Input: part model. Units: mm. Frame: model coordinates. Round coordinates to 2 decimals unless told otherwise and drop trailing zeros. Loops run counter-clockwise (first coordinate to the right, second up) from the corner with the lowest first, then second, coordinate; pieces in that order, holes last. Notation, with made-up numbers: (-10, -21) -> (45, -21) arc R33 ccw to (45, 16) -> close; hole circle Ø11 at (-39.75, 20.25). An arc over 180 degrees is marked (long way). Answer in a Markdown table with one row per item. Add a question column.
Q1. Ray query, L1, parallel to X at y = 3, z = 74 (3 decimals); L2, parallel to X at y = 4.25, z = 20; L3, parallel to X at y = 3.75, z = 33. Return the intervals inside material, ascending. Write a range as from..to.
Q2. Section A-A, the plane y = 3.75. Give the number of separate pieces and of enclosed holes in the cut face, and give its area (3 significant figures).
Q3. Section B-B, the plane z = 13. Output: boundary loops of the cut face in (x, y).
Q4. Section C-C, the plane x = 11. Output: boundary loops of the cut face in (y, z), and give its area (3 significant figures).
Q5. Section D-D, the plane z = -63. Output: boundary loops of the cut face in (x, y).
Q6. Pin query (flat end, axial travel): pin 1 (8 mm diameter, centred on x = -17, z = 57, fed in from -Y); pin 2 (2 mm diameter, centred on x = -19.05, z = -75, fed in from +Y); pin 3 (2 mm diameter, centred on y = 5.5, z = 18, fed in from +X); pin 4 (1 mm diameter, centred on y = 3, z = -15.5, fed in from -X). Return the tip coordinate at first contact, or that it passes through.
```python
from build123d import *

# Parameters (mm, degrees)
SKETCH2_R             = 90
EXTRUDE1_DEPTH        = 7
SKETCH3_R             = 8
CUT_EXTRUDE1_DEPTH    = 8
M3X0_5_TAPPED_HOLE1_D = 2.5
CIRPATTERN1_COUNT     = 4
SKETCH8_R             = 60
CUT_EXTRUDE2_DEPTH    = 8


with BuildPart() as part:
    # Sketch2 → Extrude1 (new body)
    with BuildSketch(Plane(origin=(0, 0, 0), x_dir=(1, 0, 0), z_dir=(0, 1, 0))):
        Circle(SKETCH2_R)
    extrude(amount=EXTRUDE1_DEPTH)

    # Sketch3 → Cut-Extrude1 (cut, through all)
    with BuildSketch(Plane(origin=(0, 7, 0), x_dir=(1, 0, 0), z_dir=(0, 1, 0))):
        with Locations((0, 75)):
            Circle(SKETCH3_R)
    cut_extrude1 = extrude(amount=-CUT_EXTRUDE1_DEPTH, mode=Mode.SUBTRACT)

    # M3x0.5 Tapped Hole1 (through all)
    with Locations(Plane(origin=(0, 7, 0), x_dir=(1, 0, 0), z_dir=(0, 1, 0))):
        with Locations((-19.05, 75), (19.05, 75)):
            m3x0_5_tapped_hole1 = Hole(M3X0_5_TAPPED_HOLE1_D / 2)

    # CirPattern1: Cut-Extrude1, M3x0.5 Tapped Hole1 ×4 about axis
    cirpattern1_axis = Axis((0, 0, 0), (0, 1, 0))
    for i in range(1, CIRPATTERN1_COUNT):
        add(cut_extrude1.rotate(cirpattern1_axis, i * 360 / CIRPATTERN1_COUNT), mode=Mode.SUBTRACT)
        add(m3x0_5_tapped_hole1.rotate(cirpattern1_axis, i * 360 / CIRPATTERN1_COUNT), mode=Mode.SUBTRACT)

    # Sketch8 → Cut-Extrude2 (cut, through all)
    with BuildSketch(Plane(origin=(0, 7, 0), x_dir=(1, 0, 0), z_dir=(0, 1, 0))):
        Circle(SKETCH8_R)
    extrude(amount=-CUT_EXTRUDE2_DEPTH, mode=Mode.SUBTRACT)


solid = part.part
```
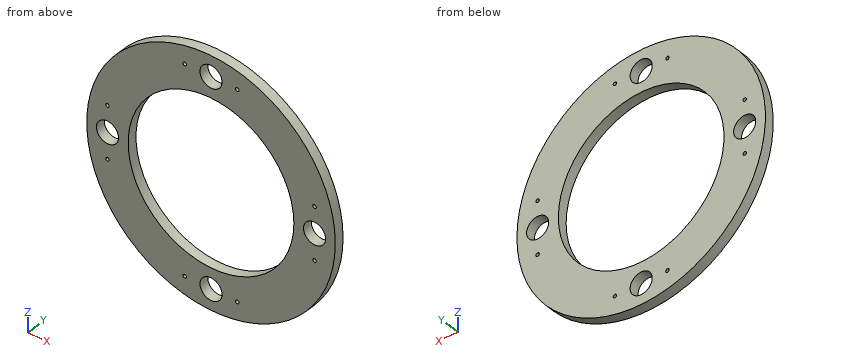
Answer block:
| question | item | result |
|---|---|---|
| 1 | L1 | -51.225..-19.8, -18.3..-7.937, 7.937..18.3, 19.8..51.225 |
| 1 | L2 | -87.75..-75.81, -74.19..-56.57, 56.57..74.19, 75.81..87.75 |
| 1 | L3 | -83.73..-50.11, 50.11..83.73 |
| 2 | separate pieces | 1 |
| 2 | enclosed holes | 13 |
| 2 | area | 13,300 mm^2 |
| 3 | outline | (-89.06, 0) -> (-58.57, 0) -> (-58.57, 7) -> (-89.06, 7) -> close; (58.57, 0) -> (89.06, 0) -> (89.06, 7) -> (58.57, 7) -> close |
| 4 | outline | (0, -89.33) -> (7, -89.33) -> (7, -58.98) -> (0, -58.98) -> close; (0, 58.98) -> (7, 58.98) -> (7, 89.33) -> (0, 89.33) -> close |
| 4 | area | 425 mm^2 |
| 5 | outline | (-64.27, 0) -> (64.27, 0) -> (64.27, 7) -> (-64.27, 7) -> close |
| 6 | pin 1 | y = 0 |
| 6 | pin 2 | through |
| 6 | pin 3 | x = 88.38 |
| 6 | pin 4 | x = -88.74 |
